Read the model definition and answer for the solid it produces. Units are mm, in the model's axes. A direction names the side the tool comes from. Give positions to 0.01 mm unless a question says otherwise; leave off trailing zeros. Order: outer loops, then holes, each group sorted by start corner. A loop starts at its lowest first (then second) coordinate and runs counter-clockwise, first axis right, second up. Notation, with made-up numbers: (88.5, 0.5) - (110.5, 0.5) arc R15 ccw to (110.5, 12.5) - close; hole circle Ø6 at (-16, 35.5). An arc over 180 degrees is marked (long way). One line per item, written item: value. Start each with the question number.
Autodesk Inventor part; units mm, degrees
ref_plane "YZ Plane" through (0, 0, 0) normal (1, 0, 0) x (0, 1, 0)
ref_plane "XZ Plane" through (0, 0, 0) normal (0, 1, 0) x (-1, 0, 0)
ref_plane "XY Plane" through (0, 0, 0) normal (0, 0, 1) x (1, 0, 0)
sketch "Sketch1" plane through (0, 0, 0) normal (1, 0, 0) x (0, 1, 0)
  line L0 (0, 10.16) -> (7.62, 10.16)
  line L1 (7.62, 10.16) -> (7.62, -10.16)
  line L2 (7.62, -10.16) -> (0, -10.16)
  line L3 (0, -10.16) -> (0, -6.35)
  line L4 (0, -6.35) -> (-2.921, -6.35)
  line L5 (-2.921, -6.35) -> (-2.921, 6.35)
  line L6 (-2.921, 6.35) -> (0, 6.35)
  line L7 (0, 6.35) -> (0, 10.16)
  point P0 (0, 0)
  dimension "d0" = 12.7
  dimension "d1" = 2.921
  dimension "d2" = 20.32
  dimension "d3" = 10.16
  dimension "d4" = 3.81
  dimension "d5" = 7.62
extrude "Extrusion1" add sketch "Sketch1" along normal blind 2.921
sketch "Sketch2" plane through (2.921, 0, 0) normal (1, 0, 0) x (0, 0, -1)
  circle A0 centre (0, 5.08) radius 1.5875
  point P0 (0, 0)
  dimension "d8" = 3.175
  dimension "d9" = 5.08
extrude "Extrusion2" cut sketch "Sketch2" against normal blind 2.921
chamfer "Chamfer1" distance 1.5875 angle 45 4 edges at (1.4605, 7.62, 10.16) (1.4605, 0, 10.16) (1.4605, 7.62, -10.16) (1.4605, 0, -10.16)
properties part number "batterywall"
1) The mould has two halves that part along Y. Classify faces 1 (the flat face through (2.921, 2, 0)), 2 (the cylindrical face through (1.481, 6.654, 0.207)), 3 (the flat face through (1.481, 0.783, 9.355)): +Y half, -Y half, draft (parallel to the pull), parting line (faces both ways), or undercut.
2) Section A-A on y = 5.08 is taken. Write down the section's boundary in (x, z), plus the area to 3 significant figures.
3) For faces 4 (the flat face through (1, -2.921, 0)), 5 (the flat face through (1, -1, -6.35)), 6 (the flat face through (1, 0, 7)), determine the directions among +Z, -Z, +X, -X, +Y, -Y from which every point of the face is accessible in a straight line to the end or side of a thin tool.
4) This flat-tipped pin is pushed along its axis until it touches: pin 1 (2.5 mm diameter, centred on y = 5.08, z = 0, fed in from -X). Where does it stop, or does it pass through?
5) Section B-B on z = 0 is taken. Write down the section's boundary in (x, y), plus the area to 3 significant figures.
6) Find the intervals of material crossed by probe 1 along Y at (x, z) = (1.15, 0); probe 2 along Z at (x, y) = (1.7, -0.75); probe 3 along Y at (x, z) = (1.35, -7.5), in increasing order. Write a range as from..to.
7) Section D-D on z = 6.75 is taken. Write down the section's boundary in (x, y), plus the area to 3 significant figures.
Solved:
1. face 1: draft
1. face 2: undercut
1. face 3: -Y half
2. outline: (0, -10.16) - (2.92, -10.16) - (2.92, -1.59) - (0, -1.59) - close; (0, 1.59) - (2.92, 1.59) - (2.92, 10.16) - (0, 10.16) - close
2. area: 50.1 mm2
3. face 4: +Z, -Z, +X, -X, -Y
3. face 5: -Z, +X, -X, -Y
3. face 6: +Z, +X, -X, -Y
4. pin 1: passes through
5. outline: (0, -2.92) - (2.92, -2.92) - (2.92, 3.49) - (0, 3.49) - close; (0, 6.67) - (2.92, 6.67) - (2.92, 7.62) - (0, 7.62) - close
5. area: 21.5 mm2
6. probe 1: y = -2.92..3.49, 6.67..7.62
6. probe 2: z = -6.35..6.35
6. probe 3: y = 0..7.62
7. outline: (0, 0) - (2.92, 0) - (2.92, 7.62) - (0, 7.62) - close
7. area: 22.3 mm2
